The figure shows three views and two pictorial views of one solid part (mm, origin at its lowest corner). Answer the questions. A direction names the side the tool comes from. Round coordinates to 2 decimals unless told otherwise and drop trailing zeros. Loops run counter-clockwise (first coordinate to the right, second up) from the corner with the lowest first, then second, coordinate; pieces in that order, holes last. Notation, with made-up numbers: (-33, 1.25) -> (-23, 1.25) arc R19 ccw to (-23, 25.25) -> close; hole circle Ø8 at (31.5, 87.25). An arc over 180 degrees is marked (long way). Use a Markdown table: item, result. Add a question column.
Q1. Given pin 1 Ø5 at (y, z) = (28.5, 4) entering from +X; pin 2 Ø12 at (y, z) = (17, 14) entering from -X; pin 3 Ø10.5 at (x, z) = (140.5, 9) entering from +Y; pin 4 Ø8 at (x, z) = (125, 10.5) entering from -Y, each flat-ended and moving along its own axis, determine where each tip first touches the part or whether it passes through.
Q2. Which of the six approach directions +Z, -Z, +X, -X, +Y, -Y give full straight-line access (tool end or side, diameter ignored) to the marked faces 4, 5 and 6?
Q3. Section A-A on y = 54 is taken. Give the vertices of the cut face in (x, z).
Q4. Section C-C on y = 31 is taken. Give the vertices of the cut face in (x, z).
Q5. Section D-D on x = 89 is taken. Give the vertices of the cut face in (y, z).
Q6. Section B-B on z = 5.25 is taken. Give the vertices of the cut face in (x, y) (1 decimal).
Q7. Consider line 1 (X direction, y = 50, z = 7.75) (1 decimal); line 2 (X direction, y = 26.5, z = 9.5); line 3 (X direction, y = 51.5, z = 16.5) (1 decimal). Determine where each line is inside the solid, lowest interval first.
Q8. For a pull along X with two mould halves and no side action, classify the marked faces 1, 2 and 3 as released by +X, released by -X, zero draft, split by the parting line, or undercut.
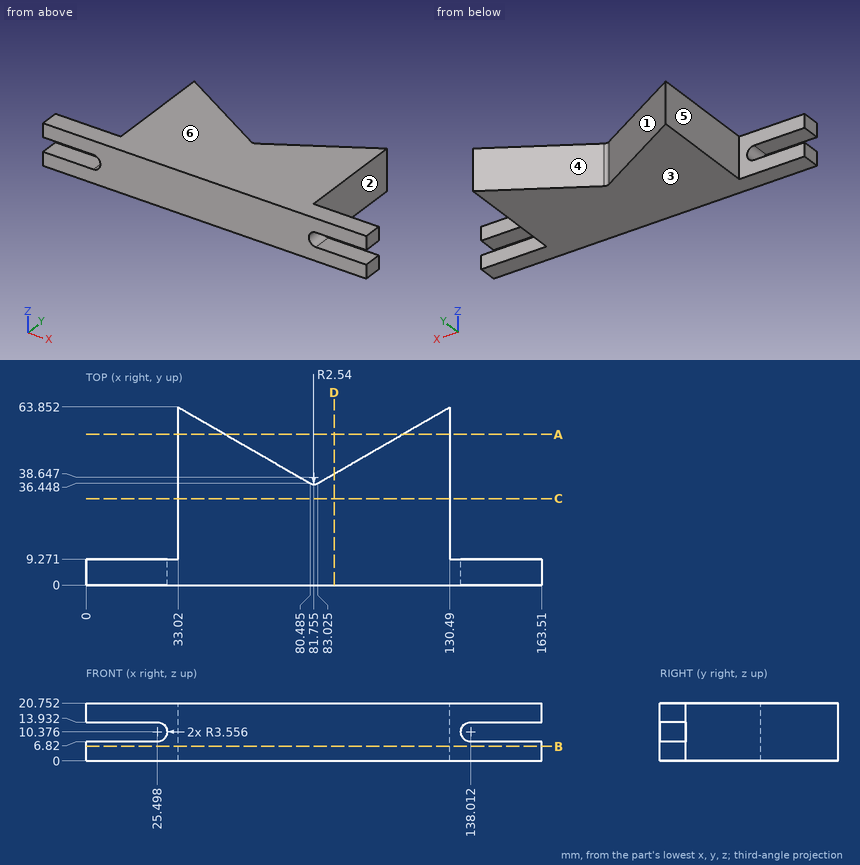
Checked values:
| question | item | result |
|---|---|---|
| 1 | pin 1 | stops at x = 130.49 |
| 1 | pin 2 | stops at x = 33.02 |
| 1 | pin 3 | stops at y = 9.27 |
| 1 | pin 4 | stops at y = 0 |
| 2 | face 4 | +Z, -Z, +Y |
| 2 | face 5 | +Z, -Z, -X, +Y |
| 2 | face 6 | +Z, +X, -X, +Y, -Y |
| 3 | outline | (33.02, 0) -> (50.08, 0) -> (50.08, 20.75) -> (33.02, 20.75) -> close; (113.43, 0) -> (130.49, 0) -> (130.49, 20.75) -> (113.43, 20.75) -> close |
| 4 | outline | (33.02, 0) -> (130.49, 0) -> (130.49, 20.75) -> (33.02, 20.75) -> close |
| 5 | outline | (0, 0) -> (39.9, 0) -> (39.9, 20.75) -> (0, 20.75) -> close |
| 6 | outline | (0, 0) -> (163.5, 0) -> (163.5, 9.3) -> (130.5, 9.3) -> (130.5, 63.9) -> (83, 36.4) arc R2.5 cw to (80.5, 36.4) -> (33, 63.9) -> (33, 9.3) -> (0, 9.3) -> close |
| 7 | line 1 | x = 33 to 57, 106.5 to 130.5 |
| 7 | line 2 | x = 33.02 to 130.49 |
| 7 | line 3 | x = 33 to 54.4, 109.1 to 130.5 |
| 8 | face 1 | undercut |
| 8 | face 2 | released by +X |
| 8 | face 3 | zero draft |
